Drawing for the job (mm, zero at the part's lowest x, y, z). A direction names the side the tool comes from. Coordinates: 2 decimals unless noted, no trailing zeros. Order: outer loops, then holes, each group sorted by start corner. A loop starts at its lowest first (then second) coordinate and runs counter-clockwise, first axis right, second up.
1) Wall check: L1, parallel to Z at x = 15.5, y = 13.5; L2, parallel to X at y = 3.5, z = 14; L3, parallel to X at y = 21, z = 6.5. Give the ranges that are in metal, low to high.
2) Cut at B-B (z = 17). List the corners of the cut face in (x, y).
3) Cut at A-A (y = 15.75). List the corners of the cut face in (x, z).
4) Cut at D-D (y = 20). List the corners of the cut face in (x, z).
5) Cut at C-C (x = 7.5). List the corners of the cut face in (y, z).
6) Pin check, flat tip, straight feed: pin 1 Ø8 at (y, z) = (11.5, 6.5) entering from -X. Stop position of the tip, or through.
7) Tool access for the marked faces 1 and 2: list every direction of +Z, -Z, +X, -X, +Y, -Y with a clear straight run to the whole face (end or side of a thin tool).
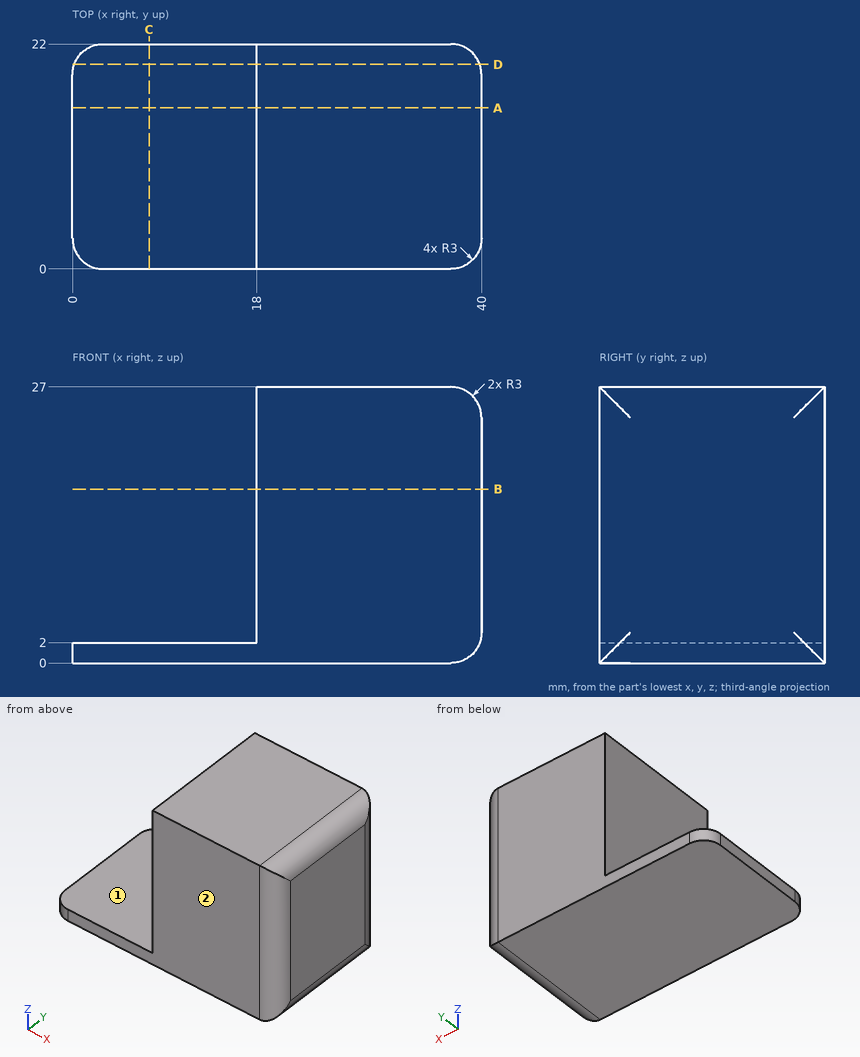
Geometry check:
1. L1: z = 0 to 2
1. L2: x = 18 to 40
1. L3: x = 18 to 39.24
2. outline: (18, 0) - (37, 0) arc R3 ccw to (40, 3) - (40, 19) arc R3 ccw to (37, 22) - (18, 22) - close
3. outline: (0, 0) - (37, 0) arc R3 ccw to (40, 3) - (40, 24) arc R3 ccw to (37, 27) - (18, 27) - (18, 2) - (0, 2) - close
4. outline: (0.17, 0) - (37, 0) arc R3 ccw to (39.83, 2) - (39.83, 25) arc R3 ccw to (37, 27) - (18, 27) - (18, 2) - (0.17, 2) - close
5. outline: (0, 0) - (22, 0) - (22, 2) - (0, 2) - close
6. pin 1: stops at x = 18
7. face 1: +Z, -X, +Y, -Y
7. face 2: +Z, -Z, +X, -X, -Y
